Verification items for the finished model (mm, model axes). A direction names the side the tool comes from. Coordinates: 2 decimals unless noted, no trailing zeros. Loops run counter-clockwise (first coordinate to the right, second up) from the corner with the lowest first, then second, coordinate; pieces in that order, holes last. Notation, with made-up numbers: (17.5, 28) -> (48.5, 28) arc R21 cw to (48.5, 32) -> close; hole circle Ø3 at (-34, 4.5). An arc over 180 degrees is marked (long way). Answer as a JSON object with one key per item and string values. Group by question number.
Q1. Set-up check for faces 1 (the flat face through (-2.5, -5, 0)), 2 (the flat face through (5, -5, -10)), 3 (the flat face through (7.5, -5, 0)): record each of +Z, -Z, +X, -X, +Y, -Y from which the full face is reachable in a straight line by a thin tool's end or side.
Q2. Cross-section at B-B on z = 25. Record the boundary of the cut face in (x, y), and give its area (3 significant figures).
Q3. Gauge pin test, flat ends, axial feed: pin 1 Ø3 at (x, z) = (9.5, 2.5) entering from -Y; pin 2 Ø5 at (y, z) = (0, -38) entering from -X; pin 3 Ø1.5 at (x, z) = (-54, 20.5) entering from +Y; pin 4 Ø6 at (x, y) = (-42.5, -5) entering from -Z. Record the tip position at first contact, or that the pin passes through.
Q4. Release check for a two-part mould opening along X. For faces 4 (the cylindrical face through (47.819, 0.342, 48.38)), 5 (the flat face through (-5, -10, 0)), 6 (the flat face through (45.543, 5.896, -46.075)) record: released by +X, released by -X, zero draft, split by the parting line, or undercut.
Q5. Scan lines: L1, parallel to Y at x = 5.85, z = -5; L2, parallel to Z at x = 11, y = 1; L3, parallel to Y at x = 11, z = -38. Record each from-to range of solid material in increasing order.
Q6. Cross-section at A-A on x = 13. Record the boundary of the cut face in (y, z).
Autodesk Inventor part; units mm, degrees
ref_plane "YZ Plane" through (0, 0, 0) normal (1, 0, 0) x (0, 1, 0)
ref_plane "XZ Plane" through (0, 0, 0) normal (0, 1, 0) x (-1, 0, 0)
ref_plane "XY Plane" through (0, 0, 0) normal (0, 0, 1) x (1, 0, 0)
sketch "스케치3" plane through (0, 0, 0) normal (0, 1, 0) x (-1, 0, 0)
  line L0 (68.3838, -28.3255) -> (28.3255, -68.3838)
  line L1 (28.3255, -68.3838) -> (-28.3255, -68.3838)
  line L2 (-28.3255, -68.3838) -> (-68.3838, -28.3255)
  line L3 (-68.3838, -28.3255) -> (-68.3838, 28.3255)
  line L4 (-68.3838, 28.3255) -> (-28.3255, 68.3838)
  line L5 (-28.3255, 68.3838) -> (28.3255, 68.3838)
  line L6 (28.3255, 68.3838) -> (68.3838, 28.3255)
  line L7 (68.3838, 28.3255) -> (68.3838, -28.3255)
  line L8 (27, -65.1838) -> (-27, -65.1838)
  line L9 (-27, -65.1838) -> (-65.1838, -27)
  line L10 (-65.1838, -27) -> (-65.1838, 27)
  line L11 (-65.1838, 27) -> (-27, 65.1838)
  line L12 (-27, 65.1838) -> (27, 65.1838)
  line L13 (27, 65.1838) -> (65.1838, 27)
  line L14 (65.1838, 27) -> (65.1838, -27)
  line L15 (65.1838, -27) -> (27, -65.1838)
  point P0 (0, 0)
  point P1 (0, 0)
  point P2 (0, 0)
  point P3 (0, 0)
  dimension "d66" = 54
  dimension "d67" = 3.2
extrude "돌출2" add sketch "스케치3" along normal blind 6.8 contours L0 L1 L2 L3 L4 L5 L6 L7 | L8 L9 L10 L11 L12 L13 L14 L15
sketch "스케치4" plane through (0, 6.8, 0) normal (0, 1, 0) x (1, 0, 0)
  line L0 (26.9172, -64.9838) -> (-26.9172, -64.9838)
  line L1 (-26.9172, -64.9838) -> (-64.9838, -26.9172)
  line L2 (-64.9838, -26.9172) -> (-64.9838, 26.9172)
  line L3 (-64.9838, 26.9172) -> (-26.9172, 64.9838)
  line L4 (-26.9172, 64.9838) -> (26.9172, 64.9838)
  line L5 (26.9172, 64.9838) -> (64.9838, 26.9172)
  line L6 (64.9838, 26.9172) -> (64.9838, -26.9172)
  line L7 (64.9838, -26.9172) -> (26.9172, -64.9838)
  line L8 (-27.6627, 66.7838) -> (27.6627, 66.7838)
  line L9 (27.6627, 66.7838) -> (66.7838, 27.6627)
  line L10 (66.7838, 27.6627) -> (66.7838, -27.6627)
  line L11 (66.7838, -27.6627) -> (27.6627, -66.7838)
  line L12 (27.6627, -66.7838) -> (-27.6627, -66.7838)
  line L13 (-27.6627, -66.7838) -> (-66.7838, -27.6627)
  line L14 (-66.7838, -27.6627) -> (-66.7838, 27.6627)
  line L15 (-66.7838, 27.6627) -> (-27.6627, 66.7838)
  line L16 (-26.8343, 64.7838) -> (26.8343, 64.7838)
  line L17 (26.8343, 64.7838) -> (64.7838, 26.8343)
  line L18 (64.7838, 26.8343) -> (64.7838, -26.8343)
  line L19 (64.7838, -26.8343) -> (26.8343, -64.7838)
  line L20 (26.8343, -64.7838) -> (-26.8343, -64.7838)
  line L21 (-26.8343, -64.7838) -> (-64.7838, -26.8343)
  line L22 (-64.7838, -26.8343) -> (-64.7838, 26.8343)
  line L23 (-64.7838, 26.8343) -> (-26.8343, 64.7838)
  line L24 (-68.3838, 28.3255) -> (-68.3838, -28.3255)
  point P0 (0, 0)
  point P1 (0, 0)
  point P2 (0, 0)
  point P3 (0, 0)
  dimension "d68" = 1.8
  dimension "d69" = 0.2
  dimension "d99" = 1.6
extrude "돌출3" cut sketch "스케치4" against normal blind 1.2 contours L0 L1 L2 L3 L4 L5 L6 L7 | L8 L9 L10 L11 L12 L13 L14 L15 | L16 L17 L18 L19 L20 L21 L22 L23
sketch "스케치9" plane through (0, 0, 0) normal (0, -1, 0) x (1, 0, 0)
  line L0 (7.5, 10) -> (2.5, 10)
  line L1 (2.5, 10) -> (2.5, -10)
  line L2 (2.5, -10) -> (7.5, -10)
  line L3 (7.5, -10) -> (7.5, 10)
  line L4 (7.5, 10) -> (2.5, -10) construction
  line L5 (2.5, 10) -> (7.5, -10) construction
  line L6 (-2.5, 10) -> (-7.5, 10)
  line L7 (-7.5, 10) -> (-7.5, -10)
  line L8 (-7.5, -10) -> (-2.5, -10)
  line L9 (-2.5, 10) -> (-7.5, -10) construction
  line L10 (-7.5, 10) -> (-2.5, -10) construction
  line L11 (-2.5, -10) -> (-2.5, 10)
  point P0 (0, 0)
  point P1 (5, 0)
  point P2 (-5, 0)
  dimension "d42" = 20
  dimension "d43" = 5
  dimension "d44" = 2.5
  dimension "d47" = 10
extrude "돌출8" add sketch "스케치9" along normal blind 10
sketch "스케치10" plane through (-7.5, 0, -10) normal (-1, 0, 0) x (0, 0, 1)
  circle A0 centre (15, -5) radius 1.25
  line L0 (19.9591, 0) -> (0.0886, 0)
  line L1 (38.3255, 0) -> (-18.3255, 0)
  circle A1 centre (5, -5) radius 1.25
  line L2 (20, 0) -> (20, -10)
  point P0 (10, 0)
  dimension "d54" = 2.5
  dimension "d57" = 10
  dimension "d62" = 5
  dimension "d63" = 5
extrude "돌출9" cut sketch "스케치10" against normal blind 20
sketch "스케치11" plane through (0, 5.6, 0) normal (0, 1, 0) x (1, 0, 0)
  line L0 (-26.8343, 64.7838) -> (26.8343, 64.7838)
  line L1 (26.8343, 64.7838) -> (64.7838, 26.8343)
  line L2 (64.7838, 26.8343) -> (64.7838, -26.8343)
  line L3 (64.7838, -26.8343) -> (26.8343, -64.7838)
  line L4 (26.8343, -64.7838) -> (-26.8343, -64.7838)
  line L5 (-26.8343, -64.7838) -> (-64.7838, -26.8343)
  line L6 (-64.7838, -26.8343) -> (-64.7838, 26.8343)
  line L7 (-64.7838, 26.8343) -> (-26.8343, 64.7838)
  line L8 (-27.6627, 66.7838) -> (27.6627, 66.7838)
  line L9 (-25.5917, 61.7838) -> (25.5917, 61.7838)
  line L10 (25.5917, 61.7838) -> (61.7838, 25.5917)
  line L11 (61.7838, 25.5917) -> (61.7838, -25.5917)
  line L12 (61.7838, -25.5917) -> (25.5917, -61.7838)
  line L13 (25.5917, -61.7838) -> (-25.5917, -61.7838)
  line L14 (-25.5917, -61.7838) -> (-61.7838, -25.5917)
  line L15 (-61.7838, -25.5917) -> (-61.7838, 25.5917)
  line L16 (-61.7838, 25.5917) -> (-25.5917, 61.7838)
  point P0 (0, 0)
  point P1 (0, 0)
  point P2 (0, 0)
  dimension "d70" = 2
  dimension "d71" = 3
extrude "돌출10" add sketch "스케치11" along normal blind 0.6 contours L0 L1 L2 L3 L4 L5 L6 L7 | L9 L10 L11 L12 L13 L14 L15 L16
fillet "모깎기1" radius 1.2 16 edges at (-48.3546, 6.8, 48.3546) (0, 6.8, 68.3838) (48.3546, 6.8, 48.3546) (68.3838, 6.8, 0) (48.3546, 6.8, -48.3546) (0, 6.8, -68.3838) (-48.3546, 6.8, -48.3546) (-68.3838, 6.8, 0) (-48.3546, 0, 48.3546) (0, 0, 68.3838) (48.3546, 0, 48.3546) (68.3838, 0, 0) (48.3546, 0, -48.3546) (0, 0, -68.3838) (-48.3546, 0, -48.3546) (-68.3838, 0, 0)
properties part number "OV-PAM_bottom_2"
Computed values:
{
 "1": {"face 1": "+Z, -Z, -Y", "face 2": "-Z, +X, -X, -Y", "face 3": "+Z, -Z, +X, -Y"},
 "2": {"outline": "(-68.38, 1.2) arc R1.2 ccw to (-67.18, 0) -> (67.18, 0) arc R1.2 ccw to (68.38, 1.2) -> (68.38, 5.6) arc R1.2 ccw to (67.18, 6.8) -> (66.78, 6.8) -> (66.78, 5.6) -> (64.78, 5.6) -> (64.78, 6.2) -> (-64.78, 6.2) -> (-64.78, 5.6) -> (-66.78, 5.6) -> (-66.78, 6.8) -> (-67.18, 6.8) arc R1.2 ccw to (-68.38, 5.6) -> close", "area": "846 mm²"},
 "3": {"pin 1": "stops at y = 0", "pin 2": "stops at x = -60.99", "pin 3": "stops at y = 6.2", "pin 4": "passes through"},
 "4": {"face 4": "released by +X", "face 5": "zero draft", "face 6": "undercut"},
 "5": {"L1": "y = -10 to -6.25, -3.75 to 6.2", "L2": "z = -68.37 to 68.37", "L3": "y = 0 to 6.2"},
 "6": {"outline": "(0, -67.18) arc R1.2 ccw to (1.2, -68.38) -> (5.6, -68.38) arc R1.2 ccw to (6.8, -67.18) -> (6.8, -66.78) -> (5.6, -66.78) -> (5.6, -64.78) -> (6.2, -64.78) -> (6.2, 64.78) -> (5.6, 64.78) -> (5.6, 66.78) -> (6.8, 66.78) -> (6.8, 67.18) arc R1.2 ccw to (5.6, 68.38) -> (1.2, 68.38) arc R1.2 ccw to (0, 67.18) -> close"}
}
